Answer from the drawing. Dimensions are ordinates in mm from the lowest x, y and z of the part. A direction names the side the tool comes from. Give positions to 0.01 mm unless a question says otherwise; leave off trailing zeros. Write each loop counter-clockwise with the first axis right and the second up, starting at its lowest first coordinate (ties: lowest second). Pieces come first, ordered by that corner, then holes. Notation, with made-up numbers: (-2, -2) -> (29, -2) arc R13 ccw to (29, 13) -> close; hole circle Ø4 at (60.5, 8.25). An arc over 180 degrees is marked (long way). Write item = value, one per line.
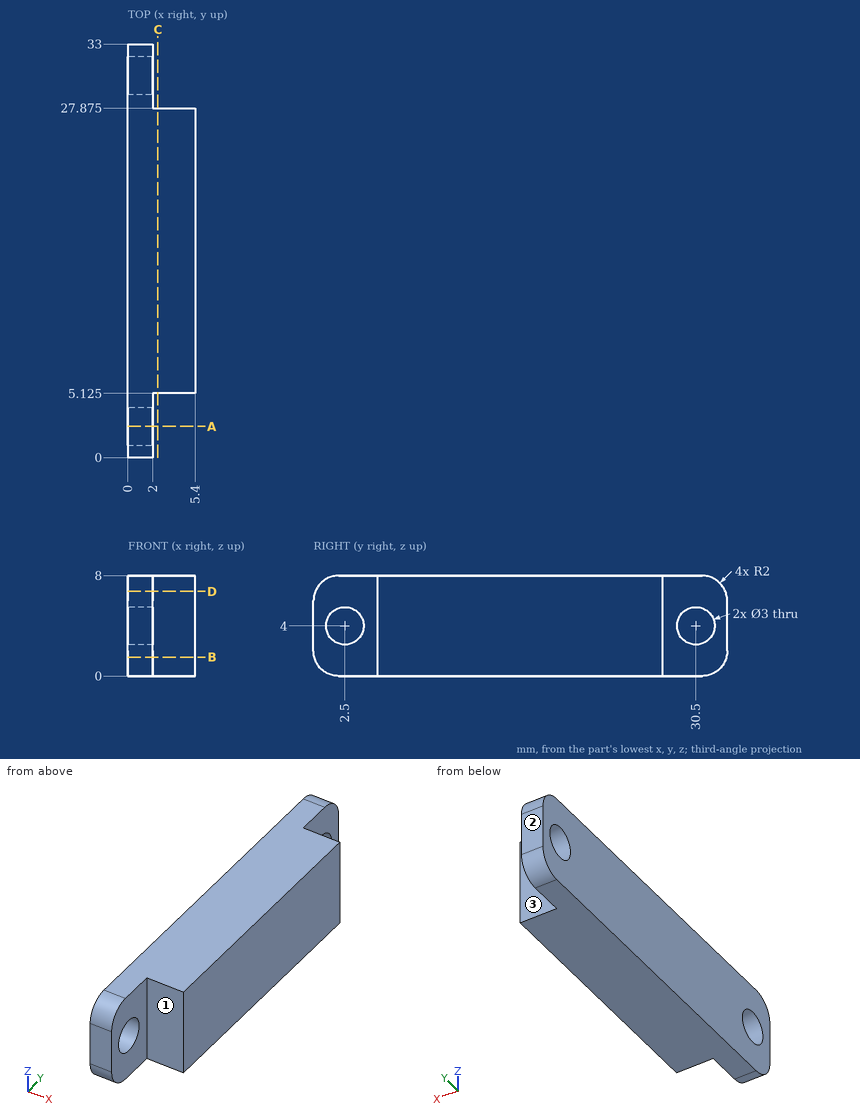
(1) The part is cut by section B-B on z = 1.5. Determine the outline of the cut face in (x, y) (1 decimal).
Checks:
outline = (0, 0.1) -> (2, 0.1) -> (2, 5.1) -> (5.4, 5.1) -> (5.4, 27.9) -> (2, 27.9) -> (2, 32.9) -> (0, 32.9) -> close
(2) The part is cut by section D-D on z = 6.75. Determine the outline of the cut face in (x, y) (3 decimals).
Checks:
outline = (0, 0.146) -> (2, 0.146) -> (2, 5.125) -> (5.4, 5.125) -> (5.4, 27.875) -> (2, 27.875) -> (2, 32.854) -> (0, 32.854) -> close
(3) Consider L1, parallel to Y at x = 1.55, z = 4.25; L2, parallel to Y at x = 0.6, z = 5; L3, parallel to Z at x = 0.6, y = 2.5. Determine where each line is inside the solid, lowest interval first.
Checks:
L1 = 0 to 1.02, 3.98 to 29.02, 31.98 to 33
L2 = 0 to 1.38, 3.62 to 29.38, 31.62 to 33
L3 = 0 to 2.5, 5.5 to 8
(4) The part is cut by section C-C on x = 2.4. Determine the outline of the cut face in (y, z) (3 decimals), plus the area to 3 significant figures.
Checks:
outline = (5.125, 0) -> (27.875, 0) -> (27.875, 8) -> (5.125, 8) -> close
area = 182 mm²
(5) The part is cut by section A-A on y = 2.5. Determine the outline of the cut face in (x, z), plus the area to 3 significant figures.
Checks:
outline = (0, 0) -> (2, 0) -> (2, 2.5) -> (0, 2.5) -> close; (0, 5.5) -> (2, 5.5) -> (2, 8) -> (0, 8) -> close
area = 10.0 mm²
(6) Given P1, Ø2.5, axis at y = 2.5, z = 4, coming from the -X side; P2, Ø4, axis at y = 2.5, z = 3.5, coming from the +X side; P3, Ø1.7, axis at x = 3.5, z = 2.5, coming from the +Y side (3 decimals), each flat-ended and moving along its own axis, determine where each tip first touches the part or whether it passes through.
Checks:
P1 = through
P2 = 2
P3 = 27.875
(7) A tool of negligible diameter and unlimited length cuts with its end or side. For the marked faces 1, 2 and 3, from which of +Z, -Z, +X, -X, +Y, -Y can it reach the whole face along a straight path? Write none if from no direction.
Checks:
face_1 = +Z, -Z, +X, -Y
face_2 = +Z, -Z, +X, -X, +Y
face_3 = +Z, -Z, +X, +Y
